from build123d import *

# Parameters (mm, degrees)
CROQUIS4_R               = 20
SALIENTE_EXTRUIR2_DEPTH  = 100
REDONDEO1_R              = 10
SALIENTE_EXTRUIR6_DEPTH  = 10
CROQUIS6_R               = 6
CROQUIS6_R_2             = 4
SALIENTE_EXTRUIR4_DEPTH  = 15
CROQUIS15_R              = 5
CORTAR_EXTRUIR5_DEPTH    = 91
CORTAR_EXTRUIR2_DEPTH    = 5
CORTAR_EXTRUIR3_DEPTH    = 5
CROQUIS12_R              = 1.5
CORTAR_EXTRUIR4_DEPTH    = 48
CROQUIS6_7_R             = 17
CROQUIS6_7_R_2           = 6
CORTAR_EXTRUIR1_DEPTH    = 10
CROQUIS6_8_R             = 20
CROQUIS6_8_R_2           = 17
SALIENTE_EXTRUIR11_DEPTH = 15


with BuildPart() as part:
    # Croquis4 → Saliente-Extruir2 (new body)
    with BuildSketch(Plane.XY):
        Circle(CROQUIS4_R)
    extrude(amount=-SALIENTE_EXTRUIR2_DEPTH)

    # Redondeo1
    redondeo1_edges = [part.edges().sort_by_distance(p)[0] for p in [
        (-20, 0, 0),
    ]]
    fillet(redondeo1_edges, radius=REDONDEO1_R)

    # Croquis8 → Saliente-Extruir6 (add)
    with BuildSketch(Plane(origin=(0, 0, 0), x_dir=(1, 0, 0), z_dir=(0, 1, 0))):
        with BuildLine():
            Line((10, 48.5), (10, 10))
            ThreePointArc((10, 10), (50, 50), (10, 90))
            Line((10, 90), (10, 51.5))
            ThreePointArc((10, 51.5), (11.5, 50), (10, 48.5))
        make_face()
    saliente_extruir6 = extrude(amount=SALIENTE_EXTRUIR6_DEPTH)

    # Croquis6 → Saliente-Extruir4 (add)
    with BuildSketch(Plane(origin=(0, 0, -100), x_dir=(-1, 0, 0), z_dir=(0, 0, -1))):
        Circle(CROQUIS6_R)
        Circle(CROQUIS6_R_2, mode=Mode.SUBTRACT)
    extrude(amount=SALIENTE_EXTRUIR4_DEPTH)

    # Simetr_a1: Saliente-Extruir6 across plane
    add(saliente_extruir6.mirror(Plane.ZX))

    # Croquis15 → Cortar-Extruir5 (cut)
    with BuildSketch(Plane.XY):
        with Locations((-12, 0)):
            Circle(CROQUIS15_R)
    extrude(amount=-CORTAR_EXTRUIR5_DEPTH, mode=Mode.SUBTRACT)

    # Croquis10 → Cortar-Extruir2 (cut)
    with BuildSketch(Plane(origin=(0, 0, 0), x_dir=(1, 0, 0), z_dir=(0, 1, 0))):
        with BuildLine():
            Line((17.320508076, 89.324421948), (17.320508076, 10.675578052))
            ThreePointArc((17.320508076, 10.675578052), (50, 50), (17.320508076, 89.324421948))
        make_face()
    cortar_extruir2 = extrude(amount=-CORTAR_EXTRUIR2_DEPTH, mode=Mode.SUBTRACT)

    # Simetr_a2: Cortar-Extruir2 across plane
    add(cortar_extruir2.mirror(Plane.ZX), mode=Mode.SUBTRACT)

    # Croquis11 → Cortar-Extruir3 (cut)
    with BuildSketch(Plane(origin=(0, 0, 0), x_dir=(1, 0, 0), z_dir=(0, 1, 0))):
        with BuildLine():
            Line((17.320508076, 89.324421948), (2.068713666, 54.962615638))
            ThreePointArc((2.068713666, 54.962615638), (1.051417021, 50.183670554), (2.052033583, 45.401205178))
            Line((2.052033583, 45.401205178), (17.320508076, 10.675578052))
            Line((17.320508076, 10.675578052), (20, 4.581515578))
            Line((20, 4.581515578), (20, 94.364916731))
            Line((20, 94.364916731), (17.320508076, 89.324421948))
        make_face()
    cortar_extruir3 = extrude(amount=-CORTAR_EXTRUIR3_DEPTH, mode=Mode.SUBTRACT)

    # Simetr_a3: Cortar-Extruir3 across plane
    add(cortar_extruir3.mirror(Plane.ZX), mode=Mode.SUBTRACT)

    # Croquis12 → Cortar-Extruir4 (cut)
    with BuildSketch(Plane(origin=(0, 0, 0), x_dir=(1, 0, 0), z_dir=(0, 1, 0))):
        with Locations((10, 50)):
            Circle(CROQUIS12_R)
        with Locations((40, 50)):
            Circle(CROQUIS12_R)
        with Locations((39.54423259, 55.20944533)):
            Circle(CROQUIS12_R)
        with Locations((38.190778624, 60.2606043)):
            Circle(CROQUIS12_R)
        with Locations((35.980762114, 65)):
            Circle(CROQUIS12_R)
        with Locations((32.981333294, 69.283628291)):
            Circle(CROQUIS12_R)
        with Locations((29.283628291, 72.981333294)):
            Circle(CROQUIS12_R)
        with Locations((25, 75.980762114)):
            Circle(CROQUIS12_R)
        with Locations((39.54423259, 44.79055467)):
            Circle(CROQUIS12_R)
        with Locations((38.190778624, 39.7393957)):
            Circle(CROQUIS12_R)
        with Locations((35.980762114, 35)):
            Circle(CROQUIS12_R)
        with Locations((32.981333294, 30.716371709)):
            Circle(CROQUIS12_R)
        with Locations((29.283628291, 27.018666706)):
            Circle(CROQUIS12_R)
        with Locations((25, 24.019237886)):
            Circle(CROQUIS12_R)
    cortar_extruir4 = extrude(amount=-CORTAR_EXTRUIR4_DEPTH, mode=Mode.SUBTRACT)

    # Croquis6_7 → Cortar-Extruir1 (cut)
    with BuildSketch(Plane(origin=(0, 0, -100), x_dir=(-1, 0, 0), z_dir=(0, 0, -1))):
        Circle(CROQUIS6_7_R)
        Circle(CROQUIS6_7_R_2, mode=Mode.SUBTRACT)
    extrude(amount=-CORTAR_EXTRUIR1_DEPTH, mode=Mode.SUBTRACT)

    # Simetr_a4: Cortar-Extruir4 across plane
    add(cortar_extruir4.mirror(Plane.ZX), mode=Mode.SUBTRACT)

    # Croquis6_8 → Saliente-Extruir11 (add)
    with BuildSketch(Plane(origin=(0, 0, -100), x_dir=(-1, 0, 0), z_dir=(0, 0, -1))):
        Circle(CROQUIS6_8_R)
        Circle(CROQUIS6_8_R_2, mode=Mode.SUBTRACT)
    extrude(amount=SALIENTE_EXTRUIR11_DEPTH)


solid = part.part
Work out the finished part from the listing and answer in its coordinate system (mm). A direction names the side the tool comes from. Round coordinates to 2 decimals unless told otherwise and drop trailing zeros. Loops run counter-clockwise (first coordinate to the right, second up) from the corner with the lowest first, then second, coordinate; pieces in that order, holes last. Notation, with made-up numbers: (56, -4.75) - (110, -4.75) arc R18 ccw to (110, 19.25) - close; hole circle Ø5 at (-4.5, 67.25). An arc over 180 degrees is marked (long way). One line per item, written item: value.
Q1. Find section C-C on z = -35. Give the vertices of the cut face in (x, y), and give its area (3 significant figures).
Check values:
outline: (6.63, -5) - (6.63, 5) - (34.48, 5) - (34.48, 10) - (17.32, 10) arc R20 ccw (long way) to (17.32, -10) - (34.48, -10) - (34.48, -5) - close; (37.48, -10) - (47.08, -10) - (47.08, -5) - (37.48, -5) - close; (37.48, 5) - (47.08, 5) - (47.08, 10) - (37.48, 10) - close; hole circle Ø10 at (-12, 0)
area: 1,300 mm2
Q2. Find section B-B on x = 25. Give the vertices of the cut face in (y, z).
Check values:
outline: (-10, -87.08) - (-5, -87.08) - (-5, -77.48) - (-10, -77.48) - close; (-10, -74.48) - (-5, -74.48) - (-5, -25.52) - (-10, -25.52) - close; (-10, -22.52) - (-5, -22.52) - (-5, -12.92) - (-10, -12.92) - close; (5, -87.08) - (10, -87.08) - (10, -77.48) - (5, -77.48) - close; (5, -74.48) - (10, -74.48) - (10, -25.52) - (5, -25.52) - close; (5, -22.52) - (10, -22.52) - (10, -12.92) - (5, -12.92) - close
Q3. Each of these flat-tipped pins is pushed along its axis until it touches: pin 1 Ø5 at (y, z) = (-9, -87.5) entering from +X; pin 2 Ø5 at (x, z) = (35.98, -65) entering from -Y; pin 3 Ø1 at (y, z) = (-15.5, -96.5) entering from -X. Where does it stop, or does it pass through?
Check values:
pin 1: x = 29.36
pin 2: y = -10
pin 3: x = -13.23
Q4. For faces 4 (the cylindrical face through (35.785, 7.465, -66.487)), 5 (the flat face through (8, 0, -90)), 6 (the flat face through (30, 10, -51)), 7 (the flat face through (25, 5, -51)), determine the directions among +Z, -Z, +X, -X, +Y, -Y from which every point of the face is accessible in a straight line to the end or side of a thin tool.
Check values:
face 4: +Y, -Y
face 5: -Z
face 6: +Z, -Z, +X, +Y
face 7: +X
Q5. Find section A-A on z = -50. Give the vertices of the cut face in (x, y), and give its area (3 significant figures).
Check values:
outline: (1.05, -5) - (1.05, 5) - (8.5, 5) - (8.5, 18.1) arc R20 ccw (long way) to (8.5, -18.1) - (8.5, -5) - close; (11.5, -16.36) arc R20 ccw to (17.32, -10) - (38.5, -10) - (38.5, -5) - (11.5, -5) - close; (11.5, 5) - (38.5, 5) - (38.5, 10) - (17.32, 10) arc R20 ccw to (11.5, 16.36) - close; (41.5, -10) - (50, -10) - (50, -5) - (41.5, -5) - close; (41.5, 5) - (50, 5) - (50, 10) - (41.5, 10) - close; hole circle Ø10 at (-12, 0)
area: 1,200 mm2
Q6. The mould has two halves that part along Y. Classify faces 1 (the flat face through (30, -10, -51)), 2 (the flat face through (9.8, 0.07, -72.38)), 3 (the cylindrical face through (34.79, -7.46, -34.09)): +Y half, -Y half, draft (parallel to the pull), parting line (faces both ways), or undercut.
Check values:
face 1: -Y half
face 2: undercut
face 3: draft
Q7. Straight lines are drawn through the part: probe 1 along Y at (x, z) = (0, -95); probe 2 along Y at (x, z) = (20, -72); probe 3 along Y at (x, z) = (-2, -102). For each, find the intervals that lie inside material, in ascending order.
Check values:
probe 1: -20 to -17, -6 to 6, 17 to 20
probe 2: -10 to -5, 5 to 10
probe 3: -19.9 to -16.88, -5.66 to -3.46, 3.46 to 5.66, 16.88 to 19.9
Q8. Find section D-D on x = 44. Give the vertices of the cut face in (y, z).
Check values:
outline: (-10, -71.07) - (-5, -71.07) - (-5, -28.93) - (-10, -28.93) - close; (5, -71.07) - (10, -71.07) - (10, -28.93) - (5, -28.93) - close
